Source: CAD feature listing. Evaluate the final solid. Frame: model axes, mm. Face numbers are marked on the shaded views. Give positions to 0.01 mm unless a question says otherwise; leave off trailing zeros. Order: outer loops, then holes, each group sorted by start corner. A loop starts at its lowest first (then second) coordinate and runs counter-clockwise, first axis right, second up. Notation, with made-up numbers: (-6.5, -13.75) - (2.5, -13.75) arc R23 ccw to (2.5, 15.25) - close; hole circle Ø8 at (37, 30.5). An arc over 180 degrees is marked (long way). Write each question's results on one line, items separated by ' | '. Start each with the question number.
Item 1: Line query: line 1 along X through (y, z) = (0.2, 0); line 2 along X through (y, z) = (2.55, -7); line 3 along Y through (x, z) = (2.5, 3). Output: solid intervals per line, ascending.
Item 2: Section B-B on z = 0. Output: boundary loops of the cut face in (x, y).
Item 3: Section C-C on y = 3.85. Output: boundary loops of the cut face in (x, z), and give its area (3 significant figures).
Item 4: Section A-A on x = 0. Output: boundary loops of the cut face in (y, z).
Item 5: Contact query for flat-ended pins moving along their axis: pin 1 Ø17 at (x, z) = (0, -7) entering from -Y; pin 2 Ø3.5 at (x, z) = (-7.75, -13.42) entering from +Y; pin 3 Ø2.5 at (x, z) = (7.75, -13.42) entering from -Y; pin 4 Ø8 at (x, z) = (-3.5, -10) entering from +Y. Output: stop coordinate, or through.
Item 6: Mould query, pull axis Z, two halves, no side actions, for the marked faces 1, 2, 3 and 4. Classes: released by +Z, released by -Z, zero draft, split by the parting line, or undercut.
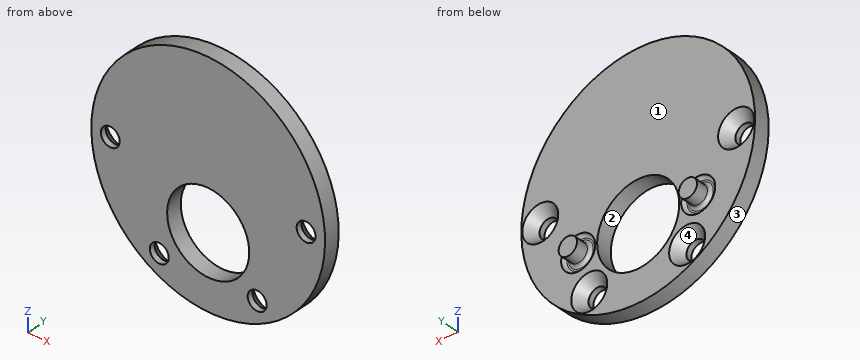
```python
from build123d import *

# Parameters (mm, degrees)
SKETCH1_R                = 18.5
SKETCH1_R_2              = 1.5
BOSS_EXTRUDE1_DEPTH      = 2.5
BOSS_EXTRUDE2_DEPTH      = 1.9
BOSS_EXTRUDE2_DEPTH_BACK = 1
SKETCH2_R                = 1.45
CUT_EXTRUDE3_START       = -0.5
SKETCH6_R                = 2.7
SKETCH6_R_2              = 1.45
CUT_EXTRUDE3_DEPTH       = 0.5
SKETCH4_R                = 6.5
CUT_EXTRUDE1_DEPTH       = 27.282123202
CHAMFER1_SIZE            = 1.35
CHAMFER1_SIZE2           = 1.6
FILLET1_R                = 0.5


with BuildPart() as part:
    # Sketch1 → Boss-Extrude1 (new body)
    with BuildSketch(Plane(origin=(0, 0, 0), x_dir=(1, 0, 0), z_dir=(0, 1, 0))):
        with Locations(Location((0, 0, 0), (0, 0, 270))):
            Circle(SKETCH1_R)
        with Locations(Location((-7.75, 13.423393759, 0), (0, 0, 270))):
            Circle(SKETCH1_R_2, mode=Mode.SUBTRACT)
        with Locations(Location((-15.5, 0, 0), (0, 0, 270))):
            Circle(SKETCH1_R_2, mode=Mode.SUBTRACT)
        with Locations(Location((7.75, 13.423393759, 0), (0, 0, 270))):
            Circle(SKETCH1_R_2, mode=Mode.SUBTRACT)
        with Locations(Location((15.5, 0, 0), (0, 0, 270))):
            Circle(SKETCH1_R_2, mode=Mode.SUBTRACT)
    extrude(amount=BOSS_EXTRUDE1_DEPTH)

    # Sketch2 → Boss-Extrude2 (add, two sides: drawn at the far end of the back side and taken through both)
    with BuildSketch(Plane(origin=(0, 2.5, 0), x_dir=(1, 0, 0), z_dir=(0, 1, 0)).offset(-BOSS_EXTRUDE2_DEPTH_BACK)):
        with Locations(Location((-9.5, 7, 0), (0, 0, 270))):
            Circle(SKETCH2_R)
        with Locations(Location((9.5, 7, 0), (0, 0, 270))):
            Circle(SKETCH2_R)
    extrude(amount=BOSS_EXTRUDE2_DEPTH + BOSS_EXTRUDE2_DEPTH_BACK)

    # Sketch6 → Cut-Extrude3 (cut)
    # profile 1 of 2: a face of its own
    with BuildSketch(Plane(origin=(0, 2.5, 0), x_dir=(1, 0, 0), z_dir=(0, 1, 0)).offset(CUT_EXTRUDE3_START)):
        with Locations(Location((-9.5, 7, 0), (0, 0, 270))):
            Circle(SKETCH6_R)
        with Locations(Location((-9.5, 7, 0), (0, 0, 270))):
            Circle(SKETCH6_R_2, mode=Mode.SUBTRACT)
    # profile 2 of 2: a face of its own
    with BuildSketch(Plane(origin=(0, 2.5, 0), x_dir=(1, 0, 0), z_dir=(0, 1, 0)).offset(CUT_EXTRUDE3_START)):
        with Locations(Location((9.5, 7, 0), (0, 0, 270))):
            Circle(SKETCH6_R)
        with Locations(Location((9.5, 7, 0), (0, 0, 270))):
            Circle(SKETCH6_R_2, mode=Mode.SUBTRACT)
    extrude(amount=CUT_EXTRUDE3_DEPTH, mode=Mode.SUBTRACT)

    # Sketch4 → Cut-Extrude1 (cut, through all)
    with BuildSketch(Plane(origin=(0, 2.5, 0), x_dir=(1, 0, 0), z_dir=(0, 1, 0))):
        with Locations(Location((0, 7, 0), (0, 0, 270))):
            Circle(SKETCH4_R)
    extrude(amount=-CUT_EXTRUDE1_DEPTH, mode=Mode.SUBTRACT)

    # Chamfer1
    chamfer1_edges = [part.edges().sort_by_distance(p)[0] for p in [
        (7.75, 2.5, -14.923393759),
        (15.5, 2.5, -1.5),
        (-7.75, 2.5, -14.923393759),
        (-15.5, 2.5, -1.5),
    ]]
    chamfer1_side = [part.faces().sort_by_distance(p)[0] for p in [
        (0, 2.5, 1.657677708),
    ]]
    chamfer(chamfer1_edges, length=CHAMFER1_SIZE, length2=CHAMFER1_SIZE2, reference=chamfer1_side[0])

    # Fillet1
    fillet1_edges = [part.edges().sort_by_distance(p)[0] for p in [
        (-9.5, 2, -9.7),
        (-9.5, 2, -8.45),
        (9.5, 2, -9.7),
        (9.5, 2, -8.45),
    ]]
    fillet(fillet1_edges, radius=FILLET1_R - 0.0001)  # a hair under: the kernel refuses the full size


solid = part.part
```
Evaluation:
1) line 1: x = -18.5 to -17, -14 to 14, 17 to 18.5 | line 2: x = -10.95 to -8.05, 8.05 to 10.95 | line 3: y = 0 to 2.5
2) outline: (-18.5, 0) - (-17, 0) - (-17, 0.9) - (-18.35, 2.5) - (-18.5, 2.5) - close; (-14, 0) - (14, 0) - (14, 0.9) - (12.65, 2.5) - (-12.65, 2.5) - (-14, 0.9) - close; (17, 0) - (18.5, 0) - (18.5, 2.5) - (18.35, 2.5) - (17, 0.9) - close
3) outline: circle Ø2.9 at (-9.5, -7); circle Ø2.9 at (9.5, -7) | area: 13.2 mm^2
4) outline: (0, -18.5) - (2.5, -18.5) - (2.5, -13.5) - (0, -13.5) - close; (0, -0.5) - (2.5, -0.5) - (2.5, 18.5) - (0, 18.5) - close
5) pin 1: stops at y = 0 | pin 2: stops at y = 1.2 | pin 3: passes through | pin 4: stops at y = 2.5
6) face 1: zero draft | face 2: undercut | face 3: split by the parting line | face 4: undercut
